Geometry: final body of the model. Coordinates: model frame, mm. A direction names the side the tool comes from. Coordinates: 2 decimals unless noted, no trailing zeros. Order: outer loops, then holes, each group sorted by start corner. A loop starts at its lowest first (then second) coordinate and runs counter-clockwise, first axis right, second up. Notation, with made-up numbers: M -7.5,72 L 34.5,72 A7 ccw 34.5,78 Z; hole C 8,-22.75 d9. An arc over 180 degrees is marked long. Use CSV: the item, a comma, the result in double quotes. Start each with the question number.
1. Pull-direction query (Z, two-part tool) for faces 6 (the flat face through (5.275, 0, -8)), 7 (the flat face through (-53.5, 0, 13)), 8 (the cylindrical face through (-46, 0, 14.2)), 9 (the flat face through (-1, 0, -5.17)); classes: pulls with the +Z half, pulls with the -Z half, needs draft (parallel to the pull), parting line crosses it, or undercut.
2. Set-up query: faces 1 (the flat face through (53.5, 0, -13)), 2 (the flat face through (15, 0, 17)), 3 (the flat face through (-8.275, 0, -8)), 4 (the flat face through (-50, 0, 15.2)), 5 (the cylindrical face through (14, 0, -14.3)). Return all of +Z, -Z, +X, -X, +Y, -Y with unobstructed straight access to the full face (end or side cutting, diameter ignored); none if empty.
3. Section query C-C on x = -46. Return the cut outline in (y, z), and give its area (3 significant figures).
4. First-contact query: P1, Ø0.9, axis at y = -0.5, z = 16, coming from the +X side. Flat tip, straight axial feed; report the tip coordinate or a pass-through.
5. Section query B-B on y = 1. State how many separate pieces and enclosed holes the cut face has, and give its area (3 significant figures).
6. Material intervals for line 1 (X direction, y = 0.55, z = 15); line 2 (Z direction, x = 14, y = 0.35); line 3 (Z direction, x = -17.5, y = 0.55), sorted ascending.
7. Section query A-A on x = 14. Return the cut outline in (y, z), and give its area (3 significant figures).
from build123d import *

# Parameters (mm, degrees)
EXTRUDE_1_DEPTH     = 1.5
SKETCH_3_R          = 3.15
CUT_EXTRUDE_2_DEPTH = 1.5
SKETCH_5_W          = 99
SKETCH_5_H          = 11.3
CUT_EXTRUDE_4_DEPTH = 10
SKETCH_6_W          = 30
SKETCH_6_H          = 3
EXTRUDE_2_DEPTH     = 3
SKETCH_8_W          = 3
SKETCH_8_H          = 18
SKETCH_8_W_2        = 4
SKETCH_8_H_2        = 30.5
EXTRUDE_3_DEPTH     = 3
SKETCH_7_R          = 1
CUT_EXTRUDE_5_DEPTH = 3


with BuildPart() as part:
    # 草图2 → 凸台-拉伸1 (new, symmetric)
    with BuildSketch(Plane(origin=(0, 0, 0), x_dir=(1, 0, 0), z_dir=(0, 1, 0))):
        Polygon((-49.5, 26.6), (-49.5, -15.2), (49.5, -15.2), (49.5, 26.599983447), align=None)
    extrude(amount=EXTRUDE_1_DEPTH, both=True)

    # 草图3 → 切除-拉伸2 (cut, symmetric)
    with BuildSketch(Plane(origin=(0, 0, 0), x_dir=(1, 0, 0), z_dir=(0, 1, 0))):
        with Locations(Location((13.999999636, 7.069989383, 0), (0, 0, 270))):
            Circle(SKETCH_3_R)
        with BuildLine():
            Line((5.275, 10.57), (5.275, 5.77))
            ThreePointArc((5.275, 5.77), (5.099264069, 5.345735931), (4.675, 5.17))
            Line((4.675, 5.17), (-7.675, 5.17))
            ThreePointArc((-7.675, 5.17), (-8.099264069, 5.345735931), (-8.275, 5.77))
            Line((-8.275, 5.77), (-8.275, 10.57))
            ThreePointArc((-8.275, 10.57), (-8.099264069, 10.994264069), (-7.675, 11.17))
            Line((-7.675, 11.17), (4.675, 11.17))
            ThreePointArc((4.675, 11.17), (5.099264069, 10.994264069), (5.275, 10.57))
        make_face()
        with BuildLine():
            Line((-13.325, 5.17), (-25.675, 5.17))
            ThreePointArc((-25.675, 5.17), (-26.099264069, 5.345735931), (-26.275, 5.77))
            Line((-26.275, 5.77), (-26.275, 10.57))
            ThreePointArc((-26.275, 10.57), (-26.099264069, 10.994264069), (-25.675, 11.17))
            Line((-25.675, 11.17), (-13.325, 11.17))
            ThreePointArc((-13.325, 11.17), (-12.900735931, 10.994264069), (-12.725, 10.57))
            Line((-12.725, 10.57), (-12.725, 5.77))
            ThreePointArc((-12.725, 5.77), (-12.900735931, 5.345735931), (-13.325, 5.17))
        make_face()
    extrude(amount=CUT_EXTRUDE_2_DEPTH, both=True, mode=Mode.SUBTRACT)

    # 草图5 → 切除-拉伸4 (cut)
    with BuildSketch(Plane.XZ.offset(1.5)):
        with Locations((0, -20.95)):
            Rectangle(SKETCH_5_W, SKETCH_5_H)
    extrude(amount=-CUT_EXTRUDE_4_DEPTH, mode=Mode.SUBTRACT)

    # 草图6 → 凸台-拉伸2 (add)
    with BuildSketch(Plane.XY.offset(15.2)):
        with Locations((30, 0)):
            Rectangle(SKETCH_6_W, SKETCH_6_H)
        with Locations((-30, 0)):
            Rectangle(SKETCH_6_W, SKETCH_6_H)
    extrude_2 = extrude(amount=EXTRUDE_2_DEPTH)

    # 镜向1: 凸台-拉伸2 across plane
    add(extrude_2.mirror(Plane.XY.offset(-0.05)))

    # 草图8 → 凸台-拉伸3 (add)
    with BuildSketch(Plane(origin=(0, 1.5, 0), x_dir=(1, 0, 0), z_dir=(0, 1, 0))):
        with Locations((-55, 0.05)):
            Rectangle(SKETCH_8_W, SKETCH_8_H)
        with Locations((-51.5, 0.05)):
            Rectangle(SKETCH_8_W_2, SKETCH_8_H_2)
        Polygon((53.5, -15.2), (53.5, -8.95), (53.5, 9.05), (53.5, 15.3), (49.5, 15.3), (49.5, -15.2), align=None)
        with Locations((55, 0.05)):
            Rectangle(SKETCH_8_W, SKETCH_8_H)
    extrude(amount=-EXTRUDE_3_DEPTH)

    # 草图7 → 切除-拉伸5 (cut)
    with BuildSketch(Plane(origin=(0, 1.5, 0), x_dir=(1, 0, 0), z_dir=(0, 1, 0))):
        with Locations((-14, 15.3)):
            Circle(SKETCH_7_R)
        with Locations((14, 15.3)):
            Circle(SKETCH_7_R)
        with Locations((46, 15.3)):
            Circle(SKETCH_7_R)
        with Locations((14, -15.2)):
            Circle(SKETCH_7_R)
        with Locations((-14, -15.2)):
            Circle(SKETCH_7_R)
        with Locations((-46, -15.2)):
            Circle(SKETCH_7_R)
        with Locations((-46, 15.3)):
            Circle(SKETCH_7_R)
        with Locations((46, -15.2)):
            Circle(SKETCH_7_R)
        with Locations((-53.5, 10.05)):
            Circle(SKETCH_7_R)
        with Locations((-53.5, -9.95)):
            Circle(SKETCH_7_R)
        with Locations((53.5, 10.05)):
            Circle(SKETCH_7_R)
        with Locations((53.5, -9.95)):
            Circle(SKETCH_7_R)
    extrude(amount=-CUT_EXTRUDE_5_DEPTH, mode=Mode.SUBTRACT)


solid = part.part
Results list:
1,face 6,"undercut"
1,face 7,"needs draft"
1,face 8,"pulls with the +Z half"
1,face 9,"undercut"
2,face 1,"-Z, +X, +Y, -Y"
2,face 2,"+Z, +Y, -Y"
2,face 3,"+Y, -Y"
2,face 4,"+Z, -X, +Y, -Y"
2,face 5,"-Z, +Y, -Y"
3,outline,"M -1.5,-14.3 L 1.5,-14.3 L 1.5,14.2 L -1.5,14.2 Z"
3,area,"85.5 mm²"
4,P1,"stops at x = 45"
5,separate pieces,"1"
5,enclosed holes,"3"
5,area,"3,520 mm²"
6,line 1,"x = -53.5 to -46.98, -45.02 to -14.98, -13.02 to 13.02, 14.98 to 45.02, 46.98 to 53.5"
6,line 2,"z = -14.3 to -10.22, -3.92 to 14.2"
6,line 3,"z = -18.3 to -11.17, -5.17 to 18.2"
7,outline,"M -1.5,-14.3 L 1.5,-14.3 L 1.5,-10.22 L -1.5,-10.22 Z; M -1.5,-3.92 L 1.5,-3.92 L 1.5,14.2 L -1.5,14.2 Z"
7,area,"66.6 mm²"
